Autodesk Inventor part; units mm, degrees
ref_plane "YZ Plane" through (0, 0, 0) normal (1, 0, 0) x (0, 1, 0)
ref_plane "XZ Plane" through (0, 0, 0) normal (0, 1, 0) x (-1, 0, 0)
ref_plane "XY Plane" through (0, 0, 0) normal (0, 0, 1) x (1, 0, 0)
sketch "Sketch1" plane through (0, 0, 0) normal (0, 1, 0) x (-1, 0, 0)
  line L0 (0, 0) -> (76.2, 0)
  line L1 (76.2, 0) -> (76.2, -304.8)
  line L2 (76.2, -304.8) -> (0, -304.8)
  line L3 (0, -304.8) -> (0, 0)
  dimension "d0" = 304.8
  dimension "d1" = 76.2
extrude "Extrusion1" add sketch "Sketch1" along normal blind 5.9995
sketch "Sketch2" plane through (0, 5.9995, 0) normal (0, 1, 0) x (1, 0, 0)
  line L0 (0, 0) -> (0, 304.8)
  line L1 (-76.2, 0) -> (0, 0)
  point P0 (-9.525, 12.7)
  point P1 (-9.525, 69.85)
  dimension "d4" = 57.15
  dimension "d5" = 9.525
  dimension "d13" = 12.7
hole "Hole1" at (-9.525, 5.9995, -12.7) at (-9.525, 5.9995, -69.85) direction (0, -1, 0) diameter 6.604 end through all
sketch "Sketch3" plane through (0, 5.9995, 0) normal (0, 1, 0) x (1, 0, 0)
  line L0 (0, 0) -> (0, 304.8)
  line L1 (-76.2, 304.8) -> (-76.2, 0)
  line L2 (0, 304.8) -> (-76.2, 304.8)
  point P0 (-9.525, 292.1)
  point P1 (-9.525, 234.95)
  point P2 (-66.675, 234.95)
  point P3 (-66.675, 292.1)
  dimension "d14" = 57.15
  dimension "d15" = 9.525
  dimension "d16" = 9.525
  dimension "d17" = 12.7
hole "Hole2" at (-9.525, 5.9995, -292.1) at (-9.525, 5.9995, -234.95) at (-66.675, 5.9995, -234.95) at (-66.675, 5.9995, -292.1) direction (0, -1, 0) diameter 6.604 end through all
sketch "Sketch4" plane through (0, 0, 0) normal (0, -1, 0) x (1, 0, 0)
  line L0 (0, -304.8) -> (-76.2, -304.8)
  line L1 (-76.2, 0) -> (0, 0)
  line L2 (-76.2, -304.8) -> (-76.2, 0)
  point P0 (-38.1, -279.4)
  point P1 (-38.1, -215.9)
  point P2 (-38.1, -152.4)
  point P3 (-38.1, -88.9)
  point P4 (-38.1, -25.4)
  dimension "d25" = 25.4
  dimension "d26" = 25.4
  dimension "d27" = 63.5
  dimension "d28" = 63.5
  dimension "d29" = 63.5
  dimension "d30" = 38.1
hole "Hole3" at (-38.1, 0, -279.4) at (-38.1, 0, -215.9) at (-38.1, 0, -152.4) at (-38.1, 0, -88.9) at (-38.1, 0, -25.4) direction (0, 1, 0) diameter 3.81 end through all
properties part number "GOES_Mount"
Geometry check sheet. Reference: the model listing, model coordinates, mm. Round coordinates to 2 decimals unless told otherwise and drop trailing zeros. Write each loop counter-clockwise with the first axis right and the second up, starting at its lowest first coordinate (ties: lowest second). Pieces come first, ordered by that corner, then holes.
Item 1: Section check A-A (z = -234.95). Record the boundary of the cut face in (x, y), plus the area to 3 significant figures.
Determined:
outline: (-76.2, 0) - (-69.98, 0) - (-69.98, 6) - (-76.2, 6) - close; (-63.37, 0) - (-12.83, 0) - (-12.83, 6) - (-63.37, 6) - close; (-6.22, 0) - (0, 0) - (0, 6) - (-6.22, 6) - close
area: 378 mm2
Item 2: Material ranges on line 1 along Z through (x, y) = (-38.1, 2.25) (3 decimals); line 2 along X through (y, z) = (4.5, -12.7); line 3 along X through (y, z) = (4, -152.4) (3 decimals), recorded low to high.
Determined:
line 1: z = -304.8 to -281.305, -277.495 to -217.805, -213.995 to -154.305, -150.495 to -90.805, -86.995 to -27.305, -23.495 to 0
line 2: x = -76.2 to -12.83, -6.22 to 0
line 3: x = -76.2 to -40.005, -36.195 to 0
Item 3: Go/stop test with a flat-tipped pin: pin 1 Ø1 at (y, z) = (3.5, -100) entering from +X. Record where the tip stops, or that it passes through.
Determined:
pin 1: stops at x = 0
Item 4: Section check B-B (z = -69.85). Record the boundary of the cut face in (x, y).
Determined:
outline: (-76.2, 0) - (-12.83, 0) - (-12.83, 6) - (-76.2, 6) - close; (-6.22, 0) - (0, 0) - (0, 6) - (-6.22, 6) - close
Item 5: Mould release check, pull along Z, two halves, no side actions. Record for faces 1 (the face through (-39, 3, -304.8)), 2 (the face through (-66.8, 3, -295.4)), 3 (the face through (-9.67, 2.96, -295.4)), 4 (the face through (0, 3, -155)): +Z half, -Z half, draft (parallel to the pull), parting line (faces both ways), or undercut.
Determined:
face 1: -Z half
face 2: undercut
face 3: undercut
face 4: draft
